Input: part model. Units: mm. Frame: model coordinates. A direction names the side the tool comes from. Give positions to 0.01 mm unless a question says otherwise; leave off trailing zeros. Order: outer loops, then holes, each group sorted by start corner. A loop starts at its lowest first (then second) coordinate and runs counter-clockwise, first axis right, second up. Notation, with made-up numbers: (-30, 55) - (5, 55) arc R19 ccw to (5, 63) - close; hole circle Ø10 at (47.25, 46.25). An arc over 180 degrees is marked (long way). Use a Markdown table: item, result.
from build123d import *

# Parameters (mm, degrees)
SKETCH_1_R      = 26
SKETCH_1_R_2    = 21
SKETCH_1_W      = 21
SKETCH_1_H      = 40
SKETCH_1_R_3    = 1.5
EXTRUDE_1_DEPTH = 4
EXTRUDE_START   = -4
SKETCH_2_R      = 21
SKETCH_2_R_2    = 13
SKETCH_2_R_3    = 2
EXTRUDE_4_DEPTH = 4
FILLET_1_R      = 3


with BuildPart() as part:
    # 草图1 → 凸台-拉伸1 (new body)
    # profile 1 of 3: a face of its own
    with BuildSketch(Plane(origin=(0, 0, 0), x_dir=(1, 0, 0), z_dir=(0, 1, 0))):
        with Locations((-30, 69)):
            Circle(SKETCH_1_R)
        with Locations(Location((-30, 69, 0), (0, 0, 270))):
            Circle(SKETCH_1_R_2, mode=Mode.SUBTRACT)
    # profile 2 of 3: a face of its own
    with BuildSketch(Plane(origin=(0, 0, 0), x_dir=(1, 0, 0), z_dir=(0, 1, 0))):
        with BuildLine():
            Line((-21, 40), (0, 40))
            Line((0, 40), (-4.218098415, 72.360587846))
            ThreePointArc((-4.218098415, 72.360587846), (-4.054581896, 70.683828791), (-4, 69))
            ThreePointArc((-4, 69), (-20.710760355, 44.716054134), (-49.362309755, 51.647739025))
            Line((-49.362309755, 51.647739025), (-21, 20))
            Line((-21, 20), (-21, 40))
        make_face()
    # profile 3 of 3: a face of its own
    with BuildSketch(Plane(origin=(0, 0, 0), x_dir=(1, 0, 0), z_dir=(0, 1, 0))):
        with Locations((-10.5, 20)):
            Rectangle(SKETCH_1_W, SKETCH_1_H)
        with Locations(Location((-15, 8, 0), (0, 0, 270))):
            Circle(SKETCH_1_R_3, mode=Mode.SUBTRACT)
        with Locations(Location((-3, 8, 0), (0, 0, 270))):
            Circle(SKETCH_1_R_3, mode=Mode.SUBTRACT)
        with Locations(Location((-3, 32, 0), (0, 0, 270))):
            Circle(SKETCH_1_R_3, mode=Mode.SUBTRACT)
        with Locations(Location((-15, 32, 0), (0, 0, 270))):
            Circle(SKETCH_1_R_3, mode=Mode.SUBTRACT)
    extrude(amount=EXTRUDE_1_DEPTH)

    # 草图2 → 凸台-拉伸4 (add)
    with BuildSketch(Plane(origin=(0, 4, 0), x_dir=(1, 0, 0), z_dir=(0, 1, 0)).offset(EXTRUDE_START)):
        with Locations((-30, 69)):
            Circle(SKETCH_2_R)
        with Locations(Location((-30, 69, 0), (0, 0, 270))):
            Circle(SKETCH_2_R_2, mode=Mode.SUBTRACT)
        with Locations(Location((-12.5, 69, 0), (0, 0, 270))):
            Circle(SKETCH_2_R_3, mode=Mode.SUBTRACT)
        with Locations(Location((-30, 51.5, 0), (0, 0, 270))):
            Circle(SKETCH_2_R_3, mode=Mode.SUBTRACT)
        with Locations(Location((-47.5, 69, 0), (0, 0, 270))):
            Circle(SKETCH_2_R_3, mode=Mode.SUBTRACT)
        with Locations(Location((-30, 86.5, 0), (0, 0, 270))):
            Circle(SKETCH_2_R_3, mode=Mode.SUBTRACT)
    extrude(amount=EXTRUDE_4_DEPTH)

    # 圆角1
    fillet_1_edges = [part.edges().sort_by_distance(p)[0] for p in [
        (0, 2, -40),
        (0, 2, 0),
        (-21, 2, 0),
        (-21, 2, -20),
    ]]
    fillet(fillet_1_edges, radius=FILLET_1_R)


solid = part.part
1. Section query C-C (y = 1.95). State how many separate pieces and enclosed holes the cut face has, then the cut area to 3 significant figures.
Response:
| item | result |
|---|---|
| separate pieces | 1 |
| enclosed holes | 9 |
| area | 2,860 mm^2 |
2. Pin query (flat end, axial travel): pin 1 (2.5 mm diameter, centred on x = -3, z = -8, fed in from +Y); pin 2 (1.2 mm diameter, centred on y = 2, z = -9, fed in from -X); pin 3 (1 mm diameter, centred on y = 2, z = -49, fed in from -X). Return the tip coordinate at first contact, or that it passes through.
Response:
| item | result |
|---|---|
| pin 1 | passes through |
| pin 2 | stops at x = -21 |
| pin 3 | stops at x = -47.44 |
3. Mould query, pull axis X, two halves, no side actions, for faces 3 (the face through (-35.76, 1.97, -36.47)), 4 (the face through (-11, 2, 0)), 5 (the face through (-11.899, 1.972, -67.092)), 6 (the face through (-14.93, 1.97, -9.5)). Classes: pulls with the +X half, pulls with the -X half, needs draft (parallel to the pull), parting line crosses it, or undercut.
Response:
| item | result |
|---|---|
| face 3 | pulls with the -X half |
| face 4 | needs draft |
| face 5 | undercut |
| face 6 | undercut |
4. Section query B-B (x = -29). Return loops of the section in (y, z).
Response:
| item | result |
|---|---|
| outline | (0, -94.98) - (4, -94.98) - (4, -88.23) - (0, -88.23) - close; (0, -84.77) - (4, -84.77) - (4, -81.96) - (0, -81.96) - close; (0, -56.04) - (4, -56.04) - (4, -53.23) - (0, -53.23) - close; (0, -49.77) - (4, -49.77) - (4, -28.93) - (0, -28.93) - close |
5. Set-up query: faces 1 (the face through (-29.428, 1.972, -81.987)), 2 (the face through (-21, 2, -11)). Return all of +Z, -Z, +X, -X, +Y, -Y with unobstructed straight access to the full face (end or side cutting, diameter ignored); none if empty.
Response:
| item | result |
|---|---|
| face 1 | +Y, -Y |
| face 2 | +Z, -X, +Y, -Y |
6. Section query A-A (z = -8). Return loops of the section in (x, y).
Response:
| item | result |
|---|---|
| outline | (-21, 0) - (-16.5, 0) - (-16.5, 4) - (-21, 4) - close; (-13.5, 0) - (-4.5, 0) - (-4.5, 4) - (-13.5, 4) - close; (-1.5, 0) - (0, 0) - (0, 4) - (-1.5, 4) - close |
7. Material intervals for line 1 along X through (y, z) = (2.45, -8); line 2 along Z through (x, y) = (-28.5, 2.95); line 3 along X through (y, z) = (2.95, -69), sorted ascending.
Response:
| item | result |
|---|---|
| line 1 | x = -21 to -16.5, -13.5 to -4.5, -1.5 to 0 |
| line 2 | z = -94.96 to -87.82, -85.18 to -81.91, -56.09 to -52.82, -50.18 to -28.37 |
| line 3 | x = -56 to -49.5, -45.5 to -43, -17 to -14.5, -10.5 to -3.78 |
8. Section query D-D (z = -86.5). Return loops of the section in (x, y), then the cut area to 3 significant figures.
Response:
| item | result |
|---|---|
| outline | (-49.23, 0) - (-32, 0) - (-32, 4) - (-49.23, 4) - close; (-28, 0) - (-10.77, 0) - (-10.77, 4) - (-28, 4) - close |
| area | 138 mm^2 |
